Design review of the part built by this model. Coordinates are the model's own, in mm. Face numbers are marked on the shaded views. Coordinates: 2 decimals unless noted, no trailing zeros. Loops run counter-clockwise (first coordinate to the right, second up) from the corner with the lowest first, then second, coordinate; pieces in that order, holes last. Notation, with made-up numbers: (-28.75, 25) -> (-6.75, 25) arc R18 ccw to (-6.75, 40) -> close; hole circle Ø7 at (64.25, 87.5). An arc over 180 degrees is marked (long way). Answer in a Markdown table with one row per item.
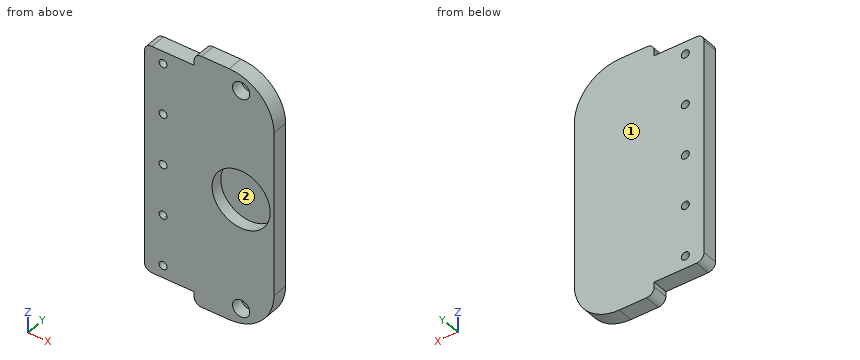
```python
from build123d import *

# Parameters (mm, degrees)
SKETCH1_W           = 52.084
SKETCH1_H           = 102.362
BOSS_EXTRUDE1_DEPTH = 6.35
SKETCH1_4_R         = 1.6
CUT_EXTRUDE2_DEPTH  = 116.026277867
SKETCH1_5_R         = 11.684
SKETCH1_5_R_2       = 3.45
CUT_EXTRUDE3_DEPTH  = 4.7625
FILLET1_R           = 18
SKETCH1_7_W         = 20
SKETCH1_7_H         = 5
CUT_EXTRUDE4_DEPTH  = 116.026277867
FILLET4_R           = 3


with BuildPart() as part:
    # Sketch1 → Boss-Extrude1 (new body)
    with BuildSketch(Plane(origin=(0, 0, 0), x_dir=(1, 0, 0), z_dir=(0, 1, 0))):
        with Locations((26.042, 51.181)):
            Rectangle(SKETCH1_W, SKETCH1_H)
    extrude(amount=BOSS_EXTRUDE1_DEPTH)

    # Sketch1<4> → Cut-Extrude2 (cut, through all)
    with BuildSketch(Plane(origin=(0, 0, 0), x_dir=(1, 0, 0), z_dir=(0, 1, 0))):
        with BuildLine():
            ThreePointArc((9.1, 71.772), (8.63137085, 72.90337085), (7.5, 73.372))
            Line((7.5, 73.372), (7.5, 70.172))
            ThreePointArc((7.5, 70.172), (8.63137085, 70.64062915), (9.1, 71.772))
        make_face()
        with BuildLine():
            Line((7.5, 70.172), (7.5, 73.372))
            ThreePointArc((7.5, 73.372), (5.9, 71.772), (7.5, 70.172))
        make_face()
        with Locations(Location((7.5, 92.362, 0), (0, 0, 270))):
            Circle(SKETCH1_4_R)
        with Locations(Location((7.5, 51.182, 0), (0, 0, 270))):
            Circle(SKETCH1_4_R)
        with Locations(Location((7.5, 30.592, 0), (0, 0, 270))):
            Circle(SKETCH1_4_R)
        with Locations(Location((7.5, 10.002, 0), (0, 0, 270))):
            Circle(SKETCH1_4_R)
    extrude(amount=CUT_EXTRUDE2_DEPTH, mode=Mode.SUBTRACT)

    # Sketch1<5> → Cut-Extrude3 (cut)
    with BuildSketch(Plane(origin=(0, 0, 0), x_dir=(1, 0, 0), z_dir=(0, 1, 0))):
        with Locations(Location((38.876, 51.18, 0), (0, 0, 90))):
            Circle(SKETCH1_5_R)
        with Locations(Location((38.876, 95.63, 0), (0, 0, 90))):
            Circle(SKETCH1_5_R_2)
        with Locations(Location((38.876, 6.73, 0), (0, 0, 90))):
            Circle(SKETCH1_5_R_2)
    extrude(amount=CUT_EXTRUDE3_DEPTH, mode=Mode.SUBTRACT)

    # Fillet1
    fillet1_edges = [part.edges().sort_by_distance(p)[0] for p in [
        (52.084, 3.175, 0),
        (52.084, 3.175, -102.362),
    ]]
    fillet(fillet1_edges, radius=FILLET1_R)

    # Sketch1<7> → Cut-Extrude4 (cut, through all)
    with BuildSketch(Plane(origin=(0, 0, 0), x_dir=(1, 0, 0), z_dir=(0, 1, 0))):
        with Locations((10, 2.5)):
            Rectangle(SKETCH1_7_W, SKETCH1_7_H)
        with Locations((10, 99.862)):
            Rectangle(SKETCH1_7_W, SKETCH1_7_H)
    extrude(amount=CUT_EXTRUDE4_DEPTH, mode=Mode.SUBTRACT)

    # Fillet4
    fillet4_edges = [part.edges().sort_by_distance(p)[0] for p in [
        (0, 3.175, -5),
        (20, 3.175, 0),
        (0, 3.175, -97.362),
        (20, 3.175, -102.362),
    ]]
    fillet(fillet4_edges, radius=FILLET4_R)


solid = part.part
```
(1) Take a section at B-B on y = 3.5. Count the separate pieces of the cut face and the enclosed holes in it, and give its area (3 significant figures).
Evaluation:
| item | result |
|---|---|
| separate pieces | 1 |
| enclosed holes | 8 |
| area | 4,440 mm² |
(2) Take a section at D-D on z = -6.73. Give the boundary of the cut face in (x, y), and give its area (3 significant figures).
Evaluation:
| item | result |
|---|---|
| outline | (0.28, 0) -> (35.43, 0) -> (35.43, 4.76) -> (42.33, 4.76) -> (42.33, 0) -> (48.12, 0) -> (48.12, 6.35) -> (0.28, 6.35) -> close |
| area | 271 mm² |
(3) To check wall thickness, follow probe 1 along Z at (x, y) = (7.5, 2); probe 2 along X at (y, z) = (1.9, -51.18); probe 3 along Z at (x, y) = (36.5, 1.75). State the ranges of each line that lie inside material, in increasing order.
Evaluation:
| item | result |
|---|---|
| probe 1 | z = -97.36 to -93.96, -90.76 to -73.37, -70.17 to -52.78, -49.58 to -32.19, -28.99 to -11.6, -8.4 to -5 |
| probe 2 | x = 0 to 5.9, 9.1 to 27.19, 50.56 to 52.08 |
| probe 3 | z = -102.2 to -98.13, -93.13 to -62.62, -39.74 to -9.23, -4.23 to -0.16 |
(4) Take a section at A-A on z = -51.18. Give the boundary of the cut face in (x, y), and give its area (3 significant figures).
Evaluation:
| item | result |
|---|---|
| outline | (0, 0) -> (5.9, 0) -> (5.9, 6.35) -> (0, 6.35) -> close; (9.1, 0) -> (27.19, 0) -> (27.19, 4.76) -> (50.56, 4.76) -> (50.56, 0) -> (52.08, 0) -> (52.08, 6.35) -> (9.1, 6.35) -> close |
| area | 199 mm² |
(5) Draft analysis for pull direction X (two halves, no side actions). For the marked faces 1 and 2, state which applies: pulls with the +X half, pulls with the -X half, needs draft (parallel to the pull), parting line crosses it, or undercut.
Evaluation:
| item | result |
|---|---|
| face 1 | needs draft |
| face 2 | undercut |
(6) For pin 1 (2 mm diameter, centred on x = 39.5, z = -7, fed in from -Y); pin 2 (10 mm diameter, centred on x = 21.5, z = -30, fed in from -Y); pin 3 (3 mm diameter, centred on x = 14.5, y = 3, fed in from -Z); pin 4 (1 mm diameter, centred on y = 2.5, z = -98.5, fed in from -X), all flat-tipped, find the tip position at first contact; note any pin that passes through.
Evaluation:
| item | result |
|---|---|
| pin 1 | stops at y = 4.76 |
| pin 2 | stops at y = 0 |
| pin 3 | stops at z = -97.36 |
| pin 4 | stops at x = 20 |
(7) Take a section at C-C on x = 48.5. Give the boundary of the cut face in (y, z).
Evaluation:
| item | result |
|---|---|
| outline | (0, -95.14) -> (6.35, -95.14) -> (6.35, -7.22) -> (0, -7.22) -> (0, -44.55) -> (4.76, -44.55) -> (4.76, -57.81) -> (0, -57.81) -> close |
